Source: CAD feature listing. Evaluate the final solid. Frame: model axes, mm. A direction names the side the tool comes from. Give positions to 0.01 mm unless a question says otherwise; leave off trailing zeros. Write each loop counter-clockwise with the first axis right and the second up, starting at its lowest first coordinate (ties: lowest second). Pieces come first, ordered by that corner, then holes. Notation, with made-up numbers: (19, 63) -> (73, 63) arc R27 ccw to (73, 81) -> close; hole circle Ø9 at (24, -6). An arc over 180 degrees is marked (long way). Use one line per item in the form item = value. Start each with the question number.
(1) Set-up query: faces 1 (the face through (240.63, 3, -1)), 2 (the face through (-70, 15.875, 0)), 3 (the face through (-64.17, 3, -1)). Return all of +Z, -Z, +X, -X, +Y, -Y with unobstructed straight access to the full face (end or side cutting, diameter ignored); none if empty.
(2) Cut plane A-A, the plane z = -5.5. Output: boundary loops of the cut face in (x, y) (3 decimals), and give its area (3 significant figures).
(3) Material intervals for line 1 along X through (y, z) = (16.25, -14); line 2 along Z through (x, y) = (-26.5, 13); line 3 along Z through (x, y) = (40, 15), sorted ascending. Write a range as from..to.
(4) First-contact query: P1, Ø1.6, axis at x = 249, y = 9.5, coming from the +Z side; P2, Ø1, axis at x = -70, y = 9, coming from the -Z side; P3, Ø4, axis at x = 246.5, z = -1.5, coming from the -Y side (3 decimals). Flat tips, straight axial feed; report the tip coordinate or a pass-through.
from build123d import *

# Parameters (mm, degrees)
F0_W     = 304.8
F0_H     = 63.5
F1_DEPTH = 19.05
F3_DEPTH = 12.7
F5_DEPTH = 12.7
F6_R     = 6.35


with BuildPart() as f1:
    # F0 (on Front) → F1 (new body)
    with BuildSketch(Plane.XZ):
        with Locations((88.229522, -0.451185)):
            Rectangle(F0_W, F0_H)
    extrude(amount=-F1_DEPTH)

    # F2 (on face) → F3 (join)
    with BuildSketch(Plane.YZ.offset(240.629522)):
        with BuildLine():
            Line((11.1252, 24.948815), (7.9248, 24.948815))
            ThreePointArc((7.9248, 24.948815), (4.566184, 23.557631), (3.175, 20.199015))
            Line((3.175, 20.199015), (3.175, -21.101385))
            ThreePointArc((3.175, -21.101385), (4.566184, -24.460001), (7.9248, -25.851185))
            Line((7.9248, -25.851185), (11.1252, -25.851185))
            ThreePointArc((11.1252, -25.851185), (14.483816, -24.460001), (15.875, -21.101385))
            Line((15.875, -21.101385), (15.875, 20.199015))
            ThreePointArc((15.875, 20.199015), (14.483816, 23.557631), (11.1252, 24.948815))
        make_face()
    extrude(amount=F3_DEPTH)

    # F4 (on face) → F5 (join)
    with BuildSketch(Plane(origin=(-64.170478, 0, 0), x_dir=(0, -1, 0), z_dir=(-1, 0, 0))):
        with BuildLine():
            Line((-7.9248, 24.948815), (-11.1252, 24.948815))
            ThreePointArc((-11.1252, 24.948815), (-14.483816, 23.557631), (-15.875, 20.199015))
            Line((-15.875, 20.199015), (-15.875, -21.101385))
            ThreePointArc((-15.875, -21.101385), (-14.483816, -24.460001), (-11.1252, -25.851185))
            Line((-11.1252, -25.851185), (-7.9248, -25.851185))
            ThreePointArc((-7.9248, -25.851185), (-4.566184, -24.460001), (-3.175, -21.101385))
            Line((-3.175, -21.101385), (-3.175, 20.199015))
            ThreePointArc((-3.175, 20.199015), (-4.566184, 23.557631), (-7.9248, 24.948815))
        make_face()
    extrude(amount=F5_DEPTH)

    # F6
    f6_edges = [f1.edges().sort_by_distance(p)[0] for p in [
        (88.229522, 0, -32.201185),
        (88.229522, 19.05, -32.201185),
    ]]
    fillet(f6_edges, radius=F6_R)


solid = f1.part
Geometry says:
q1.face_1 = +X
q1.face_2 = +Z, -Z, -X, +Y
q1.face_3 = -X
q2.outline = (-76.87, 3.175) -> (-64.17, 3.175) -> (-64.17, 0) -> (240.63, 0) -> (240.63, 3.175) -> (253.33, 3.175) -> (253.33, 15.875) -> (240.63, 15.875) -> (240.63, 19.05) -> (-64.17, 19.05) -> (-64.17, 15.875) -> (-76.87, 15.875) -> close
q2.area = 6,130 mm^2
q3.line_1 = -64.17..240.63
q3.line_2 = -32.19..31.3
q3.line_3 = -31.77..31.3
q4.P1 = 24.95
q4.P2 = -25.85
q4.P3 = 3.175
